```python
from build123d import *

# Parameters (mm, degrees)
REVOLVE1_ANGLE          = 70
CUT_EXTRUDE1_DEPTH      = 149.496943463
CUT_EXTRUDE1_DEPTH_BACK = 149.496943463
BOSS_EXTRUDE1_DEPTH     = 100
CUT_EXTRUDE2_DEPTH      = 100
CUT_EXTRUDE2_DEPTH_BACK = 100
CUT_EXTRUDE4_DEPTH      = 100


with BuildPart() as part:
    # Sketch3 → Revolve1 (revolve)
    with BuildSketch(Plane.XY):
        Polygon((0, 0), (80, 0), (80, 100), (70, 100), (30, 10), (17, 10), (17, 22.809585309), (0, 10), align=None)
    revolve(axis=Axis((80, 0, 0), (0, 1, 0)), revolution_arc=REVOLVE1_ANGLE)

    # Sketch5 → Cut-Extrude1 (cut, two sides: drawn at the far end of the back side and taken through both)
    with BuildSketch(Plane(origin=(0, 0, 0), x_dir=(1, 0, 0), z_dir=(0, 1, 0)).offset(-CUT_EXTRUDE1_DEPTH_BACK)):
        Polygon((0.205883631, -5.735764364), (71.808479557, -5.735764364), (47.318949436, -73.020195385), (2.210062516, -73.020195385), align=None)
    extrude(amount=CUT_EXTRUDE1_DEPTH + CUT_EXTRUDE1_DEPTH_BACK, mode=Mode.SUBTRACT)

    # Sketch7 → Boss-Extrude1 (add)
    with BuildSketch(Plane(origin=(0, 100, 0), x_dir=(1, 0, 0), z_dir=(0, 1, 0))):
        Polygon((71.890204546, 6.360873716), (81.890204546, -10.95963436), (78.353805314, -13.001375409), (68.353805314, 4.319132667), align=None)
    extrude(amount=-BOSS_EXTRUDE1_DEPTH)

    # Sketch8 → Cut-Extrude2 (cut, two sides: drawn at the far end of the back side and taken through both)
    with BuildSketch(Plane(origin=(0, 0, 0), x_dir=(1, 0, 0), z_dir=(0, 1, 0)).offset(-CUT_EXTRUDE2_DEPTH_BACK)):
        Polygon((71.890204546, 6.360873716), (81.890204546, -10.95963436), (87.183786138, 1.252005023), align=None)
    extrude(amount=CUT_EXTRUDE2_DEPTH + CUT_EXTRUDE2_DEPTH_BACK, mode=Mode.SUBTRACT)

    # Sketch9 → Cut-Extrude4 (cut)
    with BuildSketch(Plane(origin=(56.671992524, 0, -32.719590139), x_dir=(-0.4999999999999999, 0, -0.8660254037844387), z_dir=(0.8660254037844388, 0, -0.49999999999999994))):
        with BuildLine():
            Line((-42.376179883, 81.575757576), (-38.496668208, 81.575757576))
            Line((-38.496668208, 81.575757576), (-38.496668208, 76.289944384))
            ThreePointArc((-38.496668208, 76.289944384), (-40.436424045, 68.929279342), (-42.376179883, 76.289944384))
            Line((-42.376179883, 76.289944384), (-42.376179883, 81.575757576))
        make_face()
    extrude(amount=-CUT_EXTRUDE4_DEPTH, mode=Mode.SUBTRACT)


solid = part.part
```
Source: CAD feature listing. Evaluate the final solid. Frame: model axes, mm. A direction names the side the tool comes from. Round coordinates to 2 decimals unless told otherwise and drop trailing zeros. Order: outer loops, then holes, each group sorted by start corner. A loop starts at its lowest first (then second) coordinate and runs counter-clockwise, first axis right, second up. Notation, with made-up numbers: (88, 47.25) -> (137, 47.25) arc R22 ccw to (137, 69.25) -> close; hole circle Ø8 at (-37, 86.25). An arc over 180 degrees is marked (long way). One line per item, written item: value. Start each with the question number.
Q1. Section query C-C (y = 51). Return the cut outline in (x, z), plus the area to 3 significant figures.
Q2. Access query for faces 1 (the cylindrical face through (17.064, 16.494, 2.831)), 2 (the cylindrical face through (49.92, 4.93, 74.13)). Directions: +Z, -Z, +X, -X, +Y, -Y. A direction counts if a zero-diameter tool reaches every point of the face in a straight line with its end or side. Return the directions, or none.
Q3. Material intervals for probe 1 along Z at (x, y) = (67, 77); probe 2 along Y at (x, z) = (74.5, 3); probe 3 along X at (y, z) = (55.5, 19), sorted ascending.
Q4. Draft query along Y for faces 3 (the flat face through (74, 81.576, 4)), 4 (the flat face through (71.552, 78.97, 3.142)), 5 (the flat face through (65, 0, 25)), 6 (the flat face through (80.147, 50.7, 11.966)). Return one class per face: pulls with the +Y half, pulls with the -Y half, needs draft (parallel to the pull), parting line crosses it, or undercut.
Q5. Pin query (flat end, axial travel): pin 1 (10 mm diameter, centred on y = 79.5, z = 9.5, fed in from -X); pin 2 (6.5 mm diameter, centred on x = 21, z = 2, fed in from +Y); pin 3 (2 mm diameter, centred on y = 57.5, z = 11, fed in from -X). Return the tip coordinate at first contact, or that it passes through.
Q6. Section query A-A (y = 14.5). Return the cut outline in (x, z), plus the area to 3 significant figures.
Q7. Section query B-B (y = 36.5). Return the cut outline in (x, z), plus the area to 3 significant figures.
Findings below:
1. outline: (48.22, 0) -> (70.85, 0) -> (68.35, -4.32) -> (71.89, -6.36) -> (81.89, 10.96) -> (78.35, 13) -> (76.46, 9.72) -> (69.13, 29.86) arc R31.78 ccw to (63.92, 27.41) -> (71.81, 5.74) -> (48.74, 5.74) arc R31.78 ccw to start
1. area: 353 mm²
2. face 1: -Z, +Y
2. face 2: +Z, -X, +Y, -Y
3. probe 1: 0 to 5.74
3. probe 2: 0 to 68.97, 81.58 to 100
3. probe 3: 66.98 to 73.08
4. face 3: undercut
4. face 4: undercut
4. face 5: pulls with the -Y half
4. face 6: needs draft
5. pin 1: x = 60.24
5. pin 2: y = 10
5. pin 3: x = 69.53
6. outline: (5.97, 0) -> (17, 0) arc R63 cw to (17.26, 5.74) -> (6.19, 5.74) arc R74.03 ccw to start; (32, 0) -> (70.85, 0) -> (68.35, -4.32) -> (71.89, -6.36) -> (81.89, 10.96) -> (78.35, 13) -> (76.46, 9.72) -> (63.58, 45.11) arc R48 ccw to (58.31, 42.82) -> (71.81, 5.74) -> (32.34, 5.74) arc R48 ccw to start; (49.37, 67.39) -> (53.15, 56.99) arc R63 cw to (58.45, 59.2) -> (54.68, 69.56) arc R74.03 ccw to start
6. area: 666 mm²
7. outline: (41.78, 0) -> (70.85, 0) -> (68.35, -4.32) -> (71.89, -6.36) -> (81.89, 10.96) -> (78.35, 13) -> (76.46, 9.72) -> (66.93, 35.92) arc R38.22 ccw to (61.69, 33.55) -> (71.81, 5.74) -> (42.21, 5.74) arc R38.22 ccw to start
7. area: 427 mm²
